For this review, take the finished solid that the model builds, in its own axes (mm). A direction names the side the tool comes from. Coordinates: 2 decimals unless noted, no trailing zeros. Write each loop counter-clockwise with the first axis right and the second up, starting at its lowest first coordinate (ties: lowest second). Pieces come first, ordered by that corner, then holes. Notation, with made-up numbers: M 76,68.25 L 122,68.25 A17 ccw 122,98.25 Z; hole C 82,32 d2. An arc over 180 degrees is marked long. One line per question, with ' | ' between items.
from build123d import *

# Parameters (mm, degrees)
F0_R     = 31.75
F0_R_2   = 12.7
F1_DEPTH = 44.45
F2_R     = 127
F3_DEPTH = 3.175
F4_R     = 12.7
F5_DEPTH = 38.1
F6_R     = 127
F6_R_2   = 123.825
F7_DEPTH = 12.7


with BuildPart() as f1:
    # F0 (on Front) → F1 (new body)
    with BuildSketch(Plane.XZ):
        Circle(F0_R)
        Circle(F0_R_2, mode=Mode.SUBTRACT)
    extrude(amount=F1_DEPTH)

    # F2 (on Front) → F3 (join, symmetric)
    with BuildSketch(Plane.XZ):
        Circle(F2_R)
    extrude(amount=F3_DEPTH, both=True)

    # F4 (on face) → F5 (cut, symmetric)
    with BuildSketch(Plane.XZ.offset(3.175)):
        Circle(F4_R)
    extrude(amount=F5_DEPTH, both=True, mode=Mode.SUBTRACT)

    # F6 (on face) → F7 (cut, symmetric)
    with BuildSketch(Plane.XZ.offset(3.175)):
        Circle(F6_R)
        Circle(F6_R_2, mode=Mode.SUBTRACT)
    extrude(amount=F7_DEPTH, both=True, mode=Mode.SUBTRACT)


solid = f1.part
1) The part is to be moulded in two halves that separate along Z. For faces 1 (the cylindrical face through (-2.75, -20.97, -12.4)), 2 (the flat face through (14, -44.45, 0)), 3 (the cylindrical face through (-6.883, -23.524, -30.995)), say which applies: +Z half, -Z half, draft (parallel to the pull), parting line (faces both ways), or undercut.
Responses:
face 1: undercut | face 2: draft | face 3: parting line
2) We need section D-D on x = -95. State the section outline as (y, z) points (3 decimals).
Responses:
outline: M -3.175,-79.421 L 3.175,-79.421 L 3.175,79.421 L -3.175,79.421 Z
3) We need section B-B on x = 0. State the section outline as (y, z) points (3 decimals).
Responses:
outline: M -44.45,-31.75 L -3.175,-31.75 L -3.175,-123.825 L 3.175,-123.825 L 3.175,-12.7 L -44.45,-12.7 Z; M -44.45,12.7 L 3.175,12.7 L 3.175,123.825 L -3.175,123.825 L -3.175,31.75 L -44.45,31.75 Z
4) Insertion check: pin 1 Ø4 at (y, z) = (-26, 19.5) entering from +X; pin 2 Ø1.5 at (y, z) = (-17.5, -9) entering from -X; pin 3 Ø10 at (y, z) = (-11.5, 34) entering from -X. Each pin has a flat end and moves straight along its axis. Give the tip position at first contact, or say it passes through.
Responses:
pin 1: x = 26.49 | pin 2: x = -30.66 | pin 3: x = -12.93
5) We need section A-A on z = 0. State the section outline as (x, y) points (3 decimals), then the cut area to 3 significant figures.
Responses:
outline: M -123.825,-3.175 L -31.75,-3.175 L -31.75,-44.45 L -12.7,-44.45 L -12.7,3.175 L -123.825,3.175 Z; M 12.7,-44.45 L 31.75,-44.45 L 31.75,-3.175 L 123.825,-3.175 L 123.825,3.175 L 12.7,3.175 Z | area: 2,980 mm^2
6) We need section C-C on y = -8. State the section outline as (x, z) points, then the cut area to 3 significant figures.
Responses:
outline: C 0,0 d63.5; hole C 0,0 d25.4 | area: 2,660 mm^2
7) To check wall thickness, follow line 1 along Z through (x, y) = (0, -8); line 2 along Y through (x, z) = (-58.5, -94) (3 decimals); line 3 along X through (y, z) = (-37, 3.5). State the ranges of each line that lie inside material, in increasing order. Write a range as [from, to].
Responses:
line 1: [-31.75, -12.7], [12.7, 31.75] | line 2: [-3.175, 3.175] | line 3: [-31.56, -12.21], [12.21, 31.56]
8) Machinability: for faces 4 (the flat face through (26, 3.175, 2)), 5 (the flat face through (26, -3.175, -26)), which of the approach directions +Z, -Z, +X, -X, +Y, -Y give a long, thin tool a straight path to every point of the face, cutting with its end or side? Answer none if there is none.
Responses:
face 4: +Z, -Z, +X, -X, +Y | face 5: -Y
